```python
from build123d import *

# Parameters (mm, degrees)
F0_W     = 812.8
F0_H     = 482.6
F1_DEPTH = 1.524
F2_W     = 809.752
F2_H     = 1.524
F3_DEPTH = 482.6
F4_DEPTH = 254
F5_DEPTH = 254
F6_W     = 812.8
F6_H     = 177.8
F7_DEPTH = 1.524


with BuildPart() as f1:
    # F0 (on Top) → F1 (new body)
    with BuildSketch(Plane.XY):
        with Locations((-13.0345858634, -56.5100638679)):
            Rectangle(F0_W, F0_H)
    extrude(amount=F1_DEPTH)

    # F2 (on face) → F3 (join)
    with BuildSketch(Plane.XY.offset(1.524)):
        Polygon((393.3654141366, 184.7899361321), (391.8414141366, 184.7899361321), (391.8414141366, 183.2659361321), (391.8414141366, -296.2860638679), (391.8414141366, -297.8100638679), (393.3654141366, -297.8100638679), align=None)
        with Locations((-13.0345858634, 184.0279361321)):
            Rectangle(F2_W, F2_H)
        with Locations((-13.0345858634, -297.0480638679)):
            Rectangle(F2_W, F2_H)
        Polygon((-417.9105858634, 184.7899361321), (-419.4345858634, 184.7899361321), (-419.4345858634, -297.8100638679), (-417.9105858634, -297.8100638679), (-417.9105858634, -296.2860638679), (-417.9105858634, 183.2659361321), align=None)
    extrude(amount=F3_DEPTH)

    # F4 (add): a face of the model
    f4_faces = [f1.faces().sort_by_distance(p)[0] for p in [
        (-13.0345858634, -297.8100638679, 242.062),
    ]]
    extrude(f4_faces, amount=F4_DEPTH)

    # F5 (cut): a face of the model
    f5_faces = [f1.faces().sort_by_distance(p)[0] for p in [
        (-13.0345858634, -296.2860638679, 242.824),
    ]]
    extrude(f5_faces, amount=-F5_DEPTH, mode=Mode.SUBTRACT)

    # F6 (on face) → F7 (cut)
    with BuildSketch(Plane(origin=(0, 0, 0), x_dir=(1, 0, 0), z_dir=(0, 0, -1))):
        with Locations((-13.0345858634, 462.9100638679)):
            Rectangle(F6_W, F6_H)
    extrude(amount=-F7_DEPTH, mode=Mode.SUBTRACT)


solid = f1.part
```
Work out the finished part from the listing and answer in its coordinate system (mm). A direction names the side the tool comes from. Round coordinates to 2 decimals unless told otherwise and drop trailing zeros. Loops run counter-clockwise (first coordinate to the right, second up) from the corner with the lowest first, then second, coordinate; pieces in that order, holes last. Notation, with made-up numbers: (25, 40) -> (63, 40) arc R21 ccw to (63, 68) -> close; hole circle Ø9 at (79.25, 23). An arc over 180 degrees is marked (long way). Write each question's results on one line, items separated by ' | '. Start each with the question number.
1. Section C-C (y = 20) is taken. Determine the outline of the cut face in (x, z), plus the area to 3 significant figures.
2. Find the intervals of material crossed by probe 1 along X at (y, z) = (4, 342.5); probe 2 along Y at (x, z) = (-316.5, 185); probe 3 along Z at (x, y) = (-311.5, -62.5), in increasing order. Write a range as from..to.
3. For a pull along X with two mould halves and no side action, classify faces 1 (the face through (-419.435, -178, 239)), 2 (the face through (391.841, -178, 239)), 3 (the face through (393.365, -178, 245)) as +X half, -X half, draft (parallel to the pull), parting line (faces both ways), or undercut.
4. A tool of negligible diameter and unlimited length cuts with its end or side. For faces 4 (the face through (-19, 183.266, 239)), 5 (the face through (-19, -550.286, 239)), 6 (the face through (-19, -91, 0)), from which of +Z, -Z, +X, -X, +Y, -Y can it reach the whole face along a straight path? Write none if from no direction.
5. Section A-A (x = 247.5) is taken. Determine the outline of the cut face in (y, z), plus the area to 3 significant figures.
6. Section B-B (z = 74.5) is taken. Determine the outline of the cut face in (x, y), plus the area to 3 significant figures.
7. Given pin 1 Ø0.5 at (x, z) = (-2, 0.5) entering from -Y, flat-ended and moving along its own axis, determine where the tip first touches the part or whether it passes through.
Evaluation:
1) outline: (-419.43, 0) -> (393.37, 0) -> (393.37, 484.12) -> (391.84, 484.12) -> (391.84, 1.52) -> (-417.91, 1.52) -> (-417.91, 484.12) -> (-419.43, 484.12) -> close | area: 2,710 mm2
2) probe 1: x = -419.43..-417.91, 391.84..393.37 | probe 2: y = -551.81..-550.29, 183.27..184.79 | probe 3: z = 0..1.52
3) face 1: -X half | face 2: undercut | face 3: +X half
4) face 4: +Z | face 5: +Z, -Z | face 6: -Z, +X, -X, +Y, -Y
5) outline: (-551.81, 1.52) -> (-550.29, 1.52) -> (-550.29, 484.12) -> (-551.81, 484.12) -> close; (-374.01, 0) -> (184.79, 0) -> (184.79, 484.12) -> (183.27, 484.12) -> (183.27, 1.52) -> (-374.01, 1.52) -> close | area: 2,320 mm2
6) outline: (-419.43, -551.81) -> (393.37, -551.81) -> (393.37, 184.79) -> (-419.43, 184.79) -> close; hole (-417.91, -550.29) -> (391.84, -550.29) -> (391.84, 183.27) -> (-417.91, 183.27) -> close | area: 4,710 mm2
7) pin 1: stops at y = -374.01
